from build123d import *

# Parameters (mm, degrees)
RESSALTO_EXTRUS_O1_DEPTH = 2
ESBO_O3_R                = 2.5
RESSALTO_EXTRUS_O2_DEPTH = 2.24
ESBO_O2_R                = 0.5
CORTE_EXTRUS_O1_DEPTH    = 30.616880744
ESBO_O4_R                = 0.85
CORTE_EXTRUS_O2_DEPTH    = 30.616880744


with BuildPart() as part:
    # Esboço1 → Ressalto-extrusão1 (new body)
    with BuildSketch(Plane.XY):
        with BuildLine():
            Line((-26.705, 2.5), (26.705, 2.5))
            ThreePointArc((26.705, 2.5), (29.205, 0), (26.705, -2.5))
            Line((26.705, -2.5), (-26.705, -2.5))
            ThreePointArc((-26.705, -2.5), (-29.205, 0), (-26.705, 2.5))
        make_face()
    extrude(amount=RESSALTO_EXTRUS_O1_DEPTH)

    # Esboço3 → Ressalto-extrusão2 (add)
    with BuildSketch(Plane.XY.offset(2)):
        with Locations(Location((26.705, 0, 0), (0, 0, 90))):
            Circle(ESBO_O3_R)
    extrude(amount=RESSALTO_EXTRUS_O2_DEPTH)

    # Esboço2 → Corte-extrusão1 (cut, through all)
    with BuildSketch(Plane(origin=(0, 0, 0), x_dir=(-1, 0, 0), z_dir=(0, 0, -1))):
        with Locations((26.705, 0)):
            Circle(ESBO_O2_R)
    extrude(amount=-CORTE_EXTRUS_O1_DEPTH, mode=Mode.SUBTRACT)

    # Esboço4 → Corte-extrusão2 (cut, through all)
    with BuildSketch(Plane.XY.offset(4.24)):
        with Locations((26.705, 0)):
            Circle(ESBO_O4_R)
    extrude(amount=-CORTE_EXTRUS_O2_DEPTH, mode=Mode.SUBTRACT)


solid = part.part
Can you work these out from the model? Positions are in its coordinate system, mm. Coordinates: 2 decimals unless noted, no trailing zeros. Loops run counter-clockwise (first coordinate to the right, second up) from the corner with the lowest first, then second, coordinate; pieces in that order, holes last. Notation, with made-up numbers: (20, -35.5) - (79, -35.5) arc R27 ccw to (79, 3.5) - close; hole circle Ø3 at (30.25, 72). An arc over 180 degrees is marked (long way). Put each result on its own line as item: value. Start each with the question number.
Item 1: Suppose I cut it at A-A (y = 0). Please give me the cut outline in (x, z) (3 decimals).
Item 2: If I drill on line 1 along Z through (x, y) = (24, 2.15); line 2 along X through (y, z) = (0.15, 3.2); line 3 along X through (y, z) = (-0.4, 3.2) (3 decimals), over which ranges is the centre line in solid material (lowest first)?
Item 3: If we mould it in two halves opening along X, with no side actions, what happens to faces 1 (the face through (26.03, -0.517, 2.15)), 2 (the face through (28, 0, 4.24)), 3 (the face through (29.146, -0.542, 2.561))? For each: +X half, -X half, draft (parallel to the pull), parting line (faces both ways), or undercut.
Item 4: For pin 1 (2.5 mm diameter, centred on x = 4, y = 0.5, fed in from +Z), with a flat end and sliding along its axis, tell me the tip position at first contact or that it passes through.
Item 5: Suppose I cut it at C-C (x = 10.5). Please give me the cut outline in (y, z).
Item 6: Suppose I cut it at B-B (z = 1.3). Please give me the cut outline in (x, y) (3 decimals), and give its area (3 significant figures).
Here are the results:
1. outline: (-29.205, 0) - (-27.205, 0) - (-27.205, 2) - (-29.205, 2) - close; (-26.205, 0) - (25.855, 0) - (25.855, 4.24) - (24.205, 4.24) - (24.205, 2) - (-26.205, 2) - close; (27.555, 0) - (29.205, 0) - (29.205, 4.24) - (27.555, 4.24) - close
2. line 1: 0 to 2
2. line 2: 24.21 to 25.87, 27.54 to 29.2
2. line 3: 24.237 to 25.955, 27.455 to 29.173
3. face 1: undercut
3. face 2: draft
3. face 3: parting line
4. pin 1: z = 2
5. outline: (-2.5, 0) - (2.5, 0) - (2.5, 2) - (-2.5, 2) - close
6. outline: (-26.705, -2.5) - (26.705, -2.5) arc R2.5 ccw to (26.705, 2.5) - (-26.705, 2.5) arc R2.5 ccw to start; hole circle Ø1 at (-26.705, 0); hole circle Ø1.7 at (26.705, 0)
6. area: 284 mm²
